```python
from build123d import *

# Parameters (mm, degrees)
MAIN_PROFILE_SKETCH_W = 40
MAIN_PROFILE_SKETCH_H = 10
MAIN_PROFILE_SKETCH_R = 1.7
MAIN_EXTRUSION_DEPTH  = 3


with BuildPart() as part:
    # Main Profile Sketch → Main Extrusion (new body)
    with BuildSketch(Plane.XY.offset(44.5)):
        with Locations((-110, -36.5)):
            Rectangle(MAIN_PROFILE_SKETCH_W, MAIN_PROFILE_SKETCH_H)
        with Locations((-125, -36.5)):
            Circle(MAIN_PROFILE_SKETCH_R, mode=Mode.SUBTRACT)
        with Locations((-95, -36.5)):
            Circle(MAIN_PROFILE_SKETCH_R, mode=Mode.SUBTRACT)
    extrude(amount=-MAIN_EXTRUSION_DEPTH)


solid = part.part
```
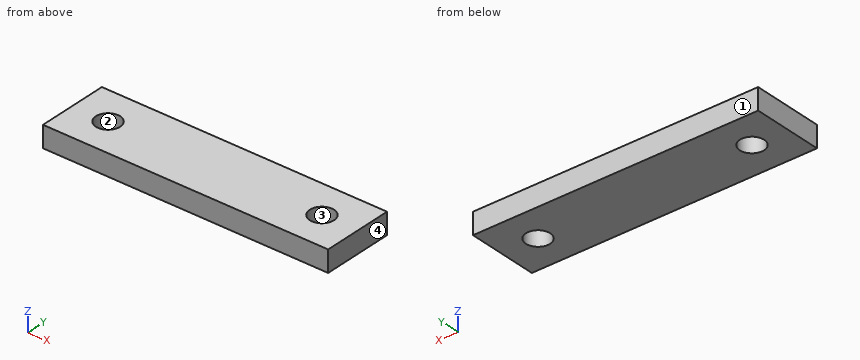
Input: part model. Units: mm. Frame: model coordinates. Face numbers are marked on the shaded views. Coordinates: 2 decimals unless noted, no trailing zeros. Write each loop counter-clockwise with the first axis right and the second up, starting at its lowest first coordinate (ties: lowest second). Pieces come first, ordered by that corner, then holes. Notation, with made-up numbers: (33, -26.75) -> (49, -26.75) arc R29 ccw to (49, 1.25) -> close; hole circle Ø1 at (28.25, 6.25). An arc over 180 degrees is marked (long way). Write each question's results on one line, items separated by ' | '.
Item 1: Section query C-C on z = 43.1. Return loops of the section in (x, y), plus the area to 3 significant figures.
Conclusion:
outline: (-130, -41.5) -> (-90, -41.5) -> (-90, -31.5) -> (-130, -31.5) -> close; hole circle Ø3.4 at (-125, -36.5); hole circle Ø3.4 at (-95, -36.5) | area: 382 mm^2
Item 2: Mould query, pull axis X, two halves, no side actions, for the marked faces 1, 2, 3 and 4. Classes: +X half, -X half, draft (parallel to the pull), parting line (faces both ways), or undercut.
Conclusion:
face 1: draft | face 2: undercut | face 3: undercut | face 4: +X half
Item 3: Pin query (flat end, axial travel): pin 1 Ø3 at (x, y) = (-96, -36.5) entering from +Z. Return the tip coordinate at first contact, or that it passes through.
Conclusion:
pin 1: stops at z = 44.5
Item 4: Material intervals for probe 1 along Y at (x, z) = (-125, 42.65); probe 2 along X at (y, z) = (-37, 43.65); probe 3 along X at (y, z) = (-35.25, 43.25), sorted ascending.
Conclusion:
probe 1: y = -41.5 to -38.2, -34.8 to -31.5 | probe 2: x = -130 to -126.62, -123.38 to -96.62, -93.38 to -90 | probe 3: x = -130 to -126.15, -123.85 to -96.15, -93.85 to -90
Item 5: Section query A-A on x = -95. Return loops of the section in (y, z), plus the area to 3 significant figures.
Conclusion:
outline: (-41.5, 41.5) -> (-38.2, 41.5) -> (-38.2, 44.5) -> (-41.5, 44.5) -> close; (-34.8, 41.5) -> (-31.5, 41.5) -> (-31.5, 44.5) -> (-34.8, 44.5) -> close | area: 19.8 mm^2
Item 6: Section query B-B on y = -36.5. Return loops of the section in (x, z).
Conclusion:
outline: (-130, 41.5) -> (-126.7, 41.5) -> (-126.7, 44.5) -> (-130, 44.5) -> close; (-123.3, 41.5) -> (-96.7, 41.5) -> (-96.7, 44.5) -> (-123.3, 44.5) -> close; (-93.3, 41.5) -> (-90, 41.5) -> (-90, 44.5) -> (-93.3, 44.5) -> close
